Answer from the drawing. Dimensions are ordinates in mm from the lowest x, y and z of the part. Coordinates: 2 decimals unless noted, no trailing zeros. Write each loop counter-clockwise with the first axis right and the second up, starting at its lowest first coordinate (ties: lowest second). Pieces come first, ordered by that corner, then holes.
1) This flat-tipped pin is pushed along its axis until it touches: pin 1 Ø3 at (x, z) = (390.5, 5.5) entering from -Y. Where does it stop, or does it pass through?
2) Find the intervals of material crossed by line 1 (Y direction, x = 207.5, z = 3.5); line 2 (Y direction, x = 427.5, z = 8); line 3 (Y direction, x = 515, z = 1.75), in increasing order.
3) The part is cut by section A-A (z = 7.75). Determine the outline of the cut face in (x, y).
4) The part is cut by section D-D (x = 310). Determine the outline of the cut face in (y, z).
5) The part is cut by section C-C (y = 40.5). Determine the outline of the cut face in (x, z), then the cut area to 3 significant figures.
6) The part is cut by section B-B (x = 398). Determine the outline of the cut face in (y, z).
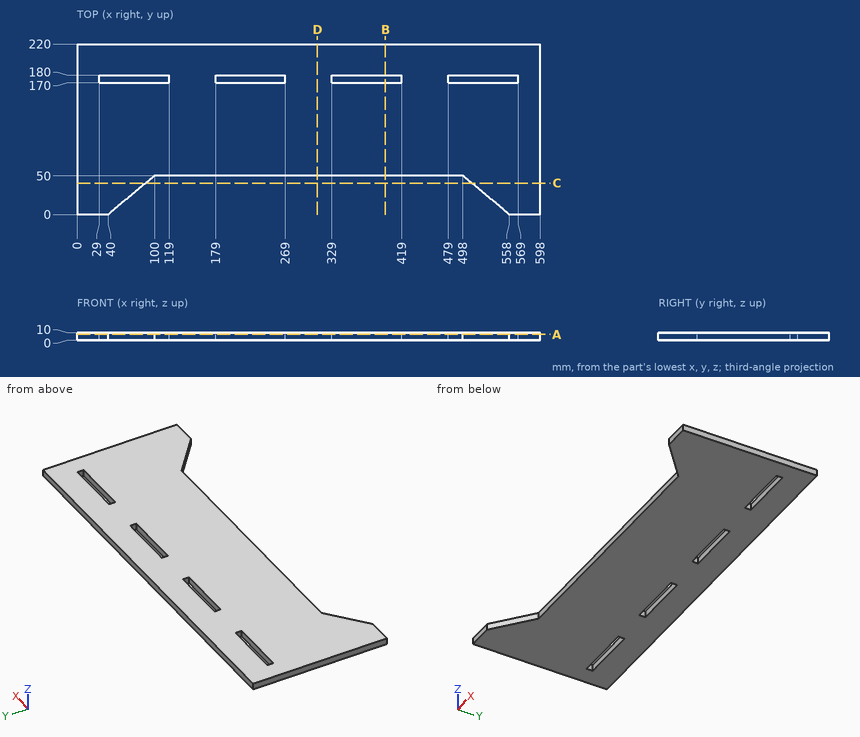
Reported:
1. pin 1: stops at y = 50
2. line 1: y = 50 to 170, 180 to 220
2. line 2: y = 50 to 220
2. line 3: y = 35.83 to 170, 180 to 220
3. outline: (0, 0) - (40, 0) - (100, 50) - (498, 50) - (558, 0) - (598, 0) - (598, 220) - (0, 220) - close; hole (29, 170) - (119, 170) - (119, 180) - (29, 180) - close; hole (179, 170) - (269, 170) - (269, 180) - (179, 180) - close; hole (329, 170) - (419, 170) - (419, 180) - (329, 180) - close; hole (479, 170) - (569, 170) - (569, 180) - (479, 180) - close
4. outline: (50, 0) - (220, 0) - (220, 10) - (50, 10) - close
5. outline: (0, 0) - (88.6, 0) - (88.6, 10) - (0, 10) - close; (509.4, 0) - (598, 0) - (598, 10) - (509.4, 10) - close
5. area: 1,770 mm2
6. outline: (50, 0) - (170, 0) - (170, 10) - (50, 10) - close; (180, 0) - (220, 0) - (220, 10) - (180, 10) - close
